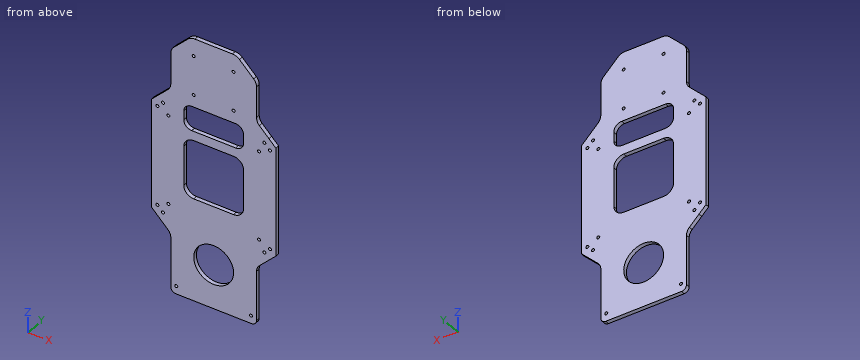
from build123d import *

# Parameters (mm, degrees)
SKETCH_1_R          = 1.5
EXTRUDE_1_DEPTH     = 4
CHAMFER_1_SIZE      = 7
SKETCH_3_W          = 60
SKETCH_3_H          = 60
SKETCH_3_R          = 1.5
SKETCH_3_R_2        = 20
SKETCH_3_H_2        = 10
SKETCH_3_H_3        = 5
CUT_EXTRUDE_1_DEPTH = 4
FILLET_3_R          = 10
FILLET_4_R          = 5
FILLET_5_R          = 8
CHAMFER_2_SIZE      = 12.5
FILLET_6_R          = 10
CHAMFER_3_SIZE      = 20
FILLET_7_R          = 10


with BuildPart() as part:
    # 草图1 → 凸台-拉伸1 (new body)
    with BuildSketch(Plane(origin=(0, 0, 0), x_dir=(1, 0, 0), z_dir=(0, 1, 0))):
        Polygon((-62.5, 62.5), (-62.5, -62.5), (-43, -62.5), (-43, -135), (43, -135), (43, -62.5), (62.5, -62.5), (62.5, 62.5), (43, 62.5), (43, 135), (-43, 135), (-43, 62.5), align=None)
        with Locations(Location((-56.5, -50.843145751, 0), (0, 0, 270))):
            Circle(SKETCH_1_R, mode=Mode.SUBTRACT)
        with Locations(Location((-50.843145751, -56.5, 0), (0, 0, 270))):
            Circle(SKETCH_1_R, mode=Mode.SUBTRACT)
        with Locations(Location((50.843145751, -56.5, 0), (0, 0, 270))):
            Circle(SKETCH_1_R, mode=Mode.SUBTRACT)
        with Locations(Location((56.5, -50.843145751, 0), (0, 0, 270))):
            Circle(SKETCH_1_R, mode=Mode.SUBTRACT)
        with Locations(Location((-56.5, 50.843145751, 0), (0, 0, 270))):
            Circle(SKETCH_1_R, mode=Mode.SUBTRACT)
        with Locations(Location((-50.843145751, 56.5, 0), (0, 0, 270))):
            Circle(SKETCH_1_R, mode=Mode.SUBTRACT)
        with Locations(Location((50.843145751, 56.5, 0), (0, 0, 270))):
            Circle(SKETCH_1_R, mode=Mode.SUBTRACT)
        with Locations(Location((56.5, 50.843145751, 0), (0, 0, 270))):
            Circle(SKETCH_1_R, mode=Mode.SUBTRACT)
        with Locations(Location((37.5, 127, 0), (0, 0, 270))):
            Circle(SKETCH_1_R, mode=Mode.SUBTRACT)
        with Locations(Location((-37.5, 127, 0), (0, 0, 270))):
            Circle(SKETCH_1_R, mode=Mode.SUBTRACT)
    extrude(amount=EXTRUDE_1_DEPTH)

    # 倒角1
    chamfer_1_edges = [part.edges().sort_by_distance(p)[0] for p in [
        (-62.5, 2, 62.5),
        (-62.5, 2, -62.5),
        (62.5, 2, -62.5),
        (62.5, 2, 62.5),
    ]]
    chamfer(chamfer_1_edges, length=CHAMFER_1_SIZE)

    # 草图3 → 切除-拉伸1 (cut)
    with BuildSketch(Plane(origin=(0, 4, 0), x_dir=(1, 0, 0), z_dir=(0, 1, 0))):
        Rectangle(SKETCH_3_W, SKETCH_3_H)
        with Locations(Location((-45.5, 45.5, 0), (0, 0, 270))):
            Circle(SKETCH_3_R)
        with Locations(Location((45.5, 45.5, 0), (0, 0, 270))):
            Circle(SKETCH_3_R)
        with Locations(Location((45.5, -45.5, 0), (0, 0, 270))):
            Circle(SKETCH_3_R)
        with Locations(Location((-45.5, -45.5, 0), (0, 0, 270))):
            Circle(SKETCH_3_R)
        with Locations(Location((0, 90, 0), (0, 0, 270))):
            Circle(SKETCH_3_R_2)
        with Locations((0, -44.5)):
            Rectangle(SKETCH_3_W, SKETCH_3_H_2)
        with Locations((0, -54.5)):
            Rectangle(SKETCH_3_W, SKETCH_3_H_2)
        with Locations((0, -62)):
            Rectangle(SKETCH_3_W, SKETCH_3_H_3)
        with Locations(Location((-20, -77, 0), (0, 0, 270))):
            Circle(SKETCH_3_R)
        with Locations(Location((20, -77, 0), (0, 0, 270))):
            Circle(SKETCH_3_R)
        with Locations(Location((20, -117, 0), (0, 0, 270))):
            Circle(SKETCH_3_R)
        with Locations(Location((-20, -117, 0), (0, 0, 270))):
            Circle(SKETCH_3_R)
    extrude(amount=-CUT_EXTRUDE_1_DEPTH, mode=Mode.SUBTRACT)

    # 圆角3
    fillet_3_edges = [part.edges().sort_by_distance(p)[0] for p in [
        (30, 2, 30),
        (-30, 2, 30),
        (-30, 2, -30),
        (30, 2, -30),
    ]]
    fillet(fillet_3_edges, radius=FILLET_3_R)

    # 圆角4
    fillet_4_edges = [part.edges().sort_by_distance(p)[0] for p in [
        (-43, 2, -135),
        (43, 2, -135),
    ]]
    fillet(fillet_4_edges, radius=FILLET_4_R)

    # 圆角5
    fillet_5_edges = [part.edges().sort_by_distance(p)[0] for p in [
        (30, 2, 39.5),
        (30, 2, 64.5),
        (-30, 2, 64.5),
        (-30, 2, 39.5),
    ]]
    fillet(fillet_5_edges, radius=FILLET_5_R)

    # 倒角2
    chamfer_2_edges = [part.edges().sort_by_distance(p)[0] for p in [
        (43, 2, -62.5),
        (-43, 2, -62.5),
        (43, 2, 62.5),
        (-43, 2, 62.5),
    ]]
    chamfer(chamfer_2_edges, length=CHAMFER_2_SIZE - 0.0001)  # a hair under: the kernel refuses the full size

    # 圆角6
    fillet_6_edges = [part.edges().sort_by_distance(p)[0] for p in [
        (43, 2, -74.9999),
        (-43, 2, -74.9999),
        (43, 2, 74.9999),
        (-43, 2, 74.9999),
    ]]
    fillet(fillet_6_edges, radius=FILLET_6_R)

    # 倒角3
    chamfer_3_edges = [part.edges().sort_by_distance(p)[0] for p in [
        (43, 2, 135),
        (-43, 2, 135),
    ]]
    chamfer(chamfer_3_edges, length=CHAMFER_3_SIZE)

    # 圆角7
    fillet_7_edges = [part.edges().sort_by_distance(p)[0] for p in [
        (43, 2, 115),
        (-23, 2, 135),
        (23, 2, 135),
        (-43, 2, 115),
    ]]
    fillet(fillet_7_edges, radius=FILLET_7_R)


solid = part.part
Here's how the part is built. I have some questions about the finished solid (model axes, mm). Give positions to 0.01 mm unless a question says otherwise; leave off trailing zeros. Write each loop counter-clockwise with the first axis right and the second up, starting at its lowest first coordinate (ties: lowest second). Pieces come first, ordered by that corner, then holes. Notation, with made-up numbers: (54, 16) -> (66, 16) arc R24 cw to (66, 29) -> close; hole circle Ø7 at (53.5, 1.25). An arc over 180 degrees is marked (long way). Use one line per item in the form item = value. Start each with the question number.
1. If I drill on L1, parallel to X at y = 3.4, z = 15.5; L2, parallel to X at y = 3.25, z = 117; L3, parallel to X at y = 1.25, z = 45.5, over which ranges is the centre line in solid material (lowest first)?
2. Imagine slicing it at A-A on z = 26. List the corners of the cut face in (x, y) for me, plus the area to 3 significant figures.
3. Imagine slicing it at C-C on z = -105.5. List the corners of the cut face in (x, y) for me.
4. Imagine slicing it at D-D on y = 1.95. State how many separate pieces and enclosed holes the cut face has, plus the area to 3 significant figures.
5. Imagine slicing it at B-B on z = 106. List the corners of the cut face in (x, y) for me, plus the area to 3 significant figures.
6. Will these pins go through, and if not, where does the flat tip stop? pin 1 Ø3 at (x, z) = (27.5, -76.5) entering from -Y; pin 2 Ø1.2 at (y, z) = (1.5, -105.5) entering from -X; pin 3 Ø2 at (y, z) = (3, -92) entering from +X.
Entries:
q1.L1 = -62.5 to -30, 30 to 62.5
q1.L2 = -40.89 to -21.5, -18.5 to 18.5, 21.5 to 40.89
q1.L3 = -62.5 to -47, -44 to -29.75, 29.75 to 44, 47 to 62.5
q2.outline = (-62.5, 0) -> (-28, 0) -> (-28, 4) -> (-62.5, 4) -> close; (28, 0) -> (62.5, 0) -> (62.5, 4) -> (28, 4) -> close
q2.area = 276 mm²
q3.outline = (-43, 0) -> (-12.64, 0) -> (-12.64, 4) -> (-43, 4) -> close; (12.64, 0) -> (43, 0) -> (43, 4) -> (12.64, 4) -> close
q4.separate_pieces = 1
q4.enclosed_holes = 21
q4.area = 21,600 mm²
q5.outline = (-43, 0) -> (43, 0) -> (43, 4) -> (-43, 4) -> close
q5.area = 344 mm²
q6.pin_1 = 0
q6.pin_2 = -43
q6.pin_3 = 43
